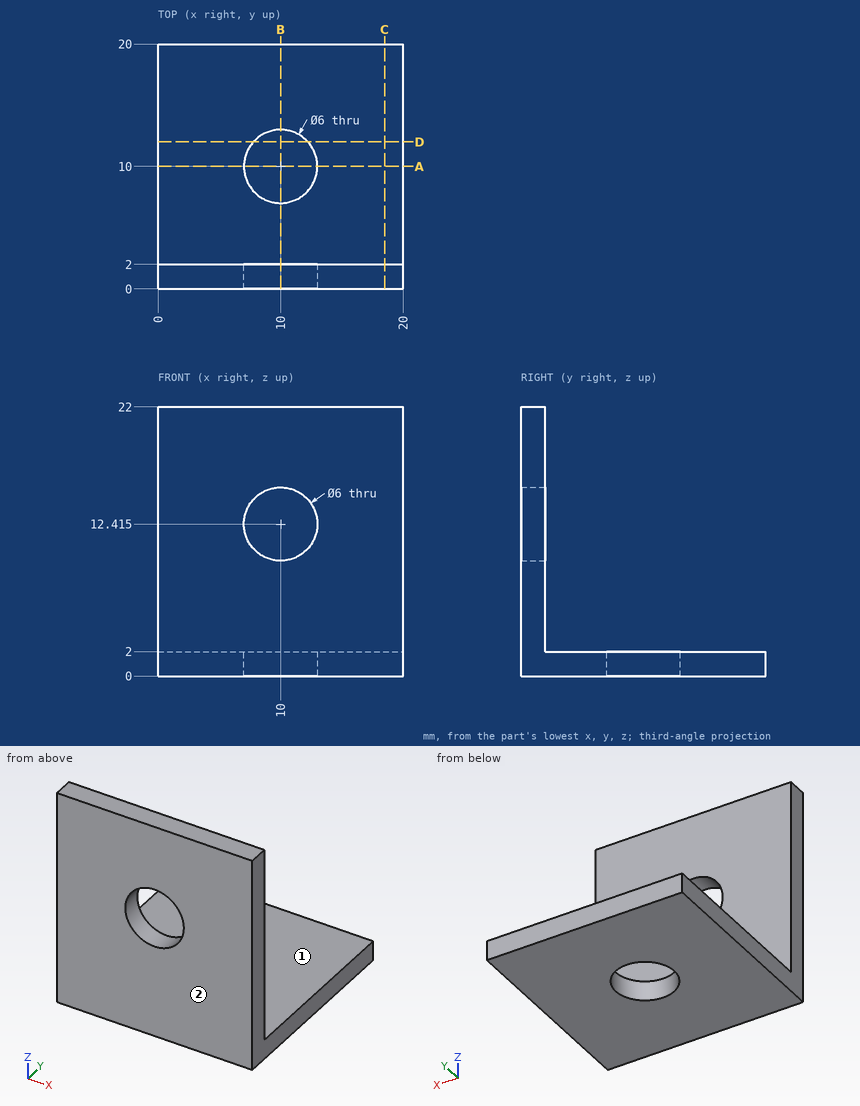
Geometry: see drawing. Coordinates: mm, zero at the bounding-box minimum. A direction names the side the tool comes from. Give positions to 0.01 mm unless a question says otherwise; leave off trailing zeros. Order: outer loops, then holes, each group sorted by start corner. A loop starts at its lowest first (then second) coordinate and runs counter-clockwise, first axis right, second up. Notation, with made-up numbers: (-6, -32) -> (4, -32) arc R22 ccw to (4, 3) -> close; hole circle Ø6 at (32, 88.5). An arc over 180 degrees is marked (long way). Write each question's results on one line, items separated by ' | '. Start each with the question number.
1) Section A-A (y = 10). Return loops of the section in (x, z).
2) Line query: line 1 (Z direction, x = 10, y = 0.55) (3 decimals); line 2 (Y direction, x = 10, z = 0.5); line 3 (Z direction, x = 3.25, y = 11.5). Output: solid intervals per line, ascending. Write a range as from..to.
3) Set-up query: the marked faces 1 and 2. Return all of +Z, -Z, +X, -X, +Y, -Y with unobstructed straight access to the full face (end or side cutting, diameter ignored); none if empty.
4) First-contact query: pin 1 (1 mm diameter, centred on x = 6, y = 13.5, fed in from -Z); pin 2 (1 mm diameter, centred on x = 3, z = 6, fed in from +Y); pin 3 (4 mm diameter, centred on x = 15.5, y = 12.5, fed in from +Z). Flat tips, straight axial feed; report the tip coordinate or a pass-through.
5) Section D-D (y = 12). Return loops of the section in (x, z).
6) Section C-C (x = 18.5). Return loops of the section in (y, z).
7) Section B-B (x = 10). Return loops of the section in (y, z) (3 decimals).
Calculated:
1) outline: (0, 0) -> (7, 0) -> (7, 2) -> (0, 2) -> close; (13, 0) -> (20, 0) -> (20, 2) -> (13, 2) -> close
2) line 1: 0..9.415, 15.415..22 | line 2: 0..7, 13..20 | line 3: 0..2
3) face 1: +Z, +X, -X, +Y | face 2: +Z, -Z, +X, -X, -Y
4) pin 1: z = 0 | pin 2: y = 2 | pin 3: z = 2
5) outline: (0, 0) -> (7.76, 0) -> (7.76, 2) -> (0, 2) -> close; (12.24, 0) -> (20, 0) -> (20, 2) -> (12.24, 2) -> close
6) outline: (0, 0) -> (20, 0) -> (20, 2) -> (2, 2) -> (2, 22) -> (0, 22) -> close
7) outline: (0, 0) -> (7, 0) -> (7, 2) -> (2, 2) -> (2, 9.415) -> (0, 9.415) -> close; (0, 15.415) -> (2, 15.415) -> (2, 22) -> (0, 22) -> close; (13, 0) -> (20, 0) -> (20, 2) -> (13, 2) -> close
